```python
from build123d import *

# Parameters (mm, degrees)
BOSS_EXTRUDE1_DEPTH = 5.64


with BuildPart() as part:
    # Sketch1 → Boss-Extrude1 (new body)
    with BuildSketch(Plane.XY):
        with BuildLine():
            Line((1246.017783232, 971.126361431), (1246.259623553, 971.126361431))
            ThreePointArc((1246.259623553, 971.126361431), (1246.966730334, 970.833468212), (1247.259623553, 970.126361431))
            Line((1247.259623553, 970.126361431), (1247.259623553, 965.277195661))
            Line((1247.259623553, 965.277195661), (1259.559623553, 965.277195661))
            Line((1259.559623553, 965.277195661), (1259.559623553, 970.126361431))
            ThreePointArc((1259.559623553, 970.126361431), (1259.852516772, 970.833468212), (1260.559623553, 971.126361431))
            Line((1260.559623553, 971.126361431), (1260.796428716, 971.126361431))
            ThreePointArc((1260.796428716, 971.126361431), (1261.403120593, 970.921298514), (1261.760992458, 970.390211362))
            Line((1261.760992458, 970.390211362), (1262.982442266, 965.92492236))
            ThreePointArc((1262.982442266, 965.92492236), (1263.115130266, 965.271220008), (1263.159623553, 964.605672702))
            Line((1263.159623553, 964.605672702), (1263.159623553, 947.021688584))
            ThreePointArc((1263.159623553, 947.021688584), (1263.130237407, 946.480395771), (1263.042424389, 945.945465561))
            Line((1263.042424389, 945.945465561), (1261.551855255, 939.182785286))
            ThreePointArc((1261.551855255, 939.182785286), (1261.201695677, 938.618528574), (1260.575295088, 938.398029891))
            Line((1260.575295088, 938.398029891), (1260.559623553, 938.398029891))
            ThreePointArc((1260.559623553, 938.398029891), (1259.852516772, 938.69092311), (1259.559623553, 939.398029891))
            Line((1259.559623553, 939.398029891), (1259.559623553, 946.477195661))
            Line((1259.559623553, 946.477195661), (1247.259623553, 946.477195661))
            Line((1247.259623553, 946.477195661), (1247.259623553, 939.398029891))
            ThreePointArc((1247.259623553, 939.398029891), (1246.966730334, 938.69092311), (1246.259623553, 938.398029891))
            Line((1246.259623553, 938.398029891), (1246.243952018, 938.398029891))
            ThreePointArc((1246.243952018, 938.398029891), (1245.617551429, 938.618528574), (1245.267391851, 939.182785286))
            Line((1245.267391851, 939.182785286), (1243.776822717, 945.945465561))
            ThreePointArc((1243.776822717, 945.945465561), (1243.689009698, 946.480395771), (1243.659623553, 947.021688584))
            Line((1243.659623553, 947.021688584), (1243.659623553, 964.732702737))
            ThreePointArc((1243.659623553, 964.732702737), (1243.706264857, 965.414052599), (1243.845318606, 966.082690842))
            Line((1243.845318606, 966.082690842), (1245.054922243, 970.396359052))
            ThreePointArc((1245.054922243, 970.396359052), (1245.413629949, 970.923229557), (1246.017783232, 971.126361431))
        make_face()
        with BuildLine():
            Line((1247.259623553, 961.277195661), (1247.259623553, 950.477195661))
            ThreePointArc((1247.259623553, 950.477195661), (1247.552516772, 949.77008888), (1248.259623553, 949.477195661))
            Line((1248.259623553, 949.477195661), (1258.559623553, 949.477195661))
            ThreePointArc((1258.559623553, 949.477195661), (1259.266730334, 949.77008888), (1259.559623553, 950.477195661))
            Line((1259.559623553, 950.477195661), (1259.559623553, 961.277195661))
            ThreePointArc((1259.559623553, 961.277195661), (1259.266730334, 961.984302442), (1258.559623553, 962.277195661))
            Line((1258.559623553, 962.277195661), (1248.259623553, 962.277195661))
            ThreePointArc((1248.259623553, 962.277195661), (1247.552516772, 961.984302442), (1247.259623553, 961.277195661))
        make_face(mode=Mode.SUBTRACT)
    extrude(amount=BOSS_EXTRUDE1_DEPTH)


solid = part.part
```
The model under review builds one solid part; all positions refer to its coordinate system, in mm. A direction names the side the tool comes from. Round coordinates to 2 decimals unless told otherwise and drop trailing zeros. Loops run counter-clockwise (first coordinate to the right, second up) from the corner with the lowest first, then second, coordinate; pieces in that order, holes last. Notation, with made-up numbers: (1, -22.75) -> (42, -22.75) arc R16 cw to (42, -16.75) -> close; hole circle Ø1 at (-11.75, 80). An arc over 180 degrees is marked (long way). Answer in a Markdown table with one row per item.
1) For pin 1 Ø1 at (x, z) = (1259.5, 3) entering from -Y; pin 2 Ø1.7 at (y, z) = (941.5, 4) entering from -X; pin 3 Ø8 at (x, y) = (1256, 957) entering from -Z; pin 4 Ø1.7 at (y, z) = (943, 3) entering from +X, all flat-tipped, find the tip position at first contact; note any pin that passes through.
Taken from the geometry:
| item | result |
|---|---|
| pin 1 | stops at y = 938.57 |
| pin 2 | stops at x = 1244.57 |
| pin 3 | stops at z = 0 |
| pin 4 | stops at x = 1262.58 |
2) Consider section A-A, the plane x = 1256.25. Write out the cut boundary in (y, z), plus the area to 3 significant figures.
Taken from the geometry:
| item | result |
|---|---|
| outline | (946.48, 0) -> (949.48, 0) -> (949.48, 5.64) -> (946.48, 5.64) -> close; (962.28, 0) -> (965.28, 0) -> (965.28, 5.64) -> (962.28, 5.64) -> close |
| area | 33.8 mm² |
3) Draft analysis for pull direction X (two halves, no side actions). For faces 6 (the cylindrical face through (1261.209, 938.624, 2.781)), 7 (the cylindrical face through (1243.705, 965.405, 2.781)), 8 (the cylindrical face through (1259.845, 970.826, 2.781)), 9 (the flat face through (1247.26, 943, 3)), state which applies: pulls with the +X half, pulls with the -X half, needs draft (parallel to the pull), parting line crosses it, or undercut.
Taken from the geometry:
| item | result |
|---|---|
| face 6 | pulls with the +X half |
| face 7 | pulls with the -X half |
| face 8 | undercut |
| face 9 | undercut |
4) Tool access review of faces 1 (the cylindrical face through (1245.41, 970.92, 2.78)), 2 (the flat face through (1263.16, 956, 3)), 3 (the cylindrical face through (1259.259, 949.762, 2.781)), 4 (the cylindrical face through (1247, 970.8, 2.8)), 5 (the flat face through (1259.56, 943, 3)): name each direction out of +Z, -Z, +X, -X, +Y, -Y from which nothing blocks a thin tool from reaching the whole face with its end or side.
Taken from the geometry:
| item | result |
|---|---|
| face 1 | +Z, -Z, -X, +Y |
| face 2 | +Z, -Z, +X, +Y, -Y |
| face 3 | +Z, -Z |
| face 4 | +Z, -Z, +Y |
| face 5 | +Z, -Z, -Y |
5) Consider section B-B, the plane y = 951.5. Write out the cut boundary in (x, z), plus the area to 3 significant figures.
Taken from the geometry:
| item | result |
|---|---|
| outline | (1243.66, 0) -> (1247.26, 0) -> (1247.26, 5.64) -> (1243.66, 5.64) -> close; (1259.56, 0) -> (1263.16, 0) -> (1263.16, 5.64) -> (1259.56, 5.64) -> close |
| area | 40.6 mm² |
6) Wall thickness on line 1 along X through (y, z) = (961, 0.85); line 2 along Y through (x, z) = (1256, 4.7); line 3 along X through (y, z) = (944.5, 4.35): over which ranges is each line inside the solid? List them lowest first.
Taken from the geometry:
| item | result |
|---|---|
| line 1 | x = 1243.66 to 1247.26, 1259.56 to 1263.16 |
| line 2 | y = 946.48 to 949.48, 962.28 to 965.28 |
| line 3 | x = 1244.1 to 1247.26, 1259.56 to 1262.72 |
